Drawing for the job (mm, zero at the part's lowest x, y, z). Give positions to 0.01 mm unless a question says otherwise; leave off trailing zeros. Write each loop counter-clockwise with the first axis right and the second up, starting at its lowest first coordinate (ties: lowest second). Pieces come first, ordered by that corner, then holes.
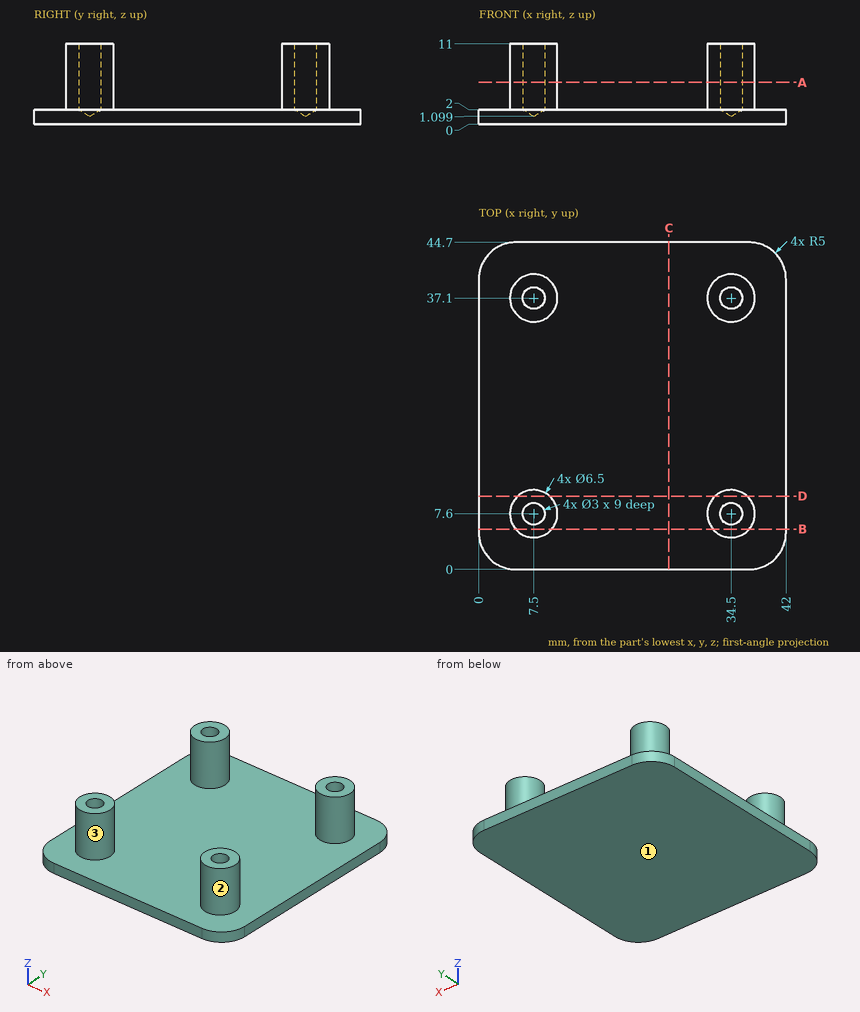
1. Probe probe 1 along Y at (x, z) = (34.5, 4.5); probe 2 along Z at (x, y) = (32.5, 24.5); probe 3 along X at (y, z) = (5, 4.5). List the from-to ranges inside material, lowest first.
Calculated:
probe 1: y = 4.35 to 6.1, 9.1 to 10.85, 33.85 to 35.6, 38.6 to 40.35
probe 2: z = 0 to 2
probe 3: x = 5.55 to 9.45, 32.55 to 36.45
2. Pull direction Y, two halves, no side cores. Call the marked faces 1, 2 and 3: +Y half, -Y half, draft (parallel to the pull), parting line (faces both ways), or undercut.
Calculated:
face 1: draft
face 2: undercut
face 3: undercut
3. Slice it at D-D, the plane y = 10. Write the cut outline in (x, z).
Calculated:
outline: (0, 0) - (42, 0) - (42, 2) - (36.69, 2) - (36.69, 11) - (32.31, 11) - (32.31, 2) - (9.69, 2) - (9.69, 11) - (5.31, 11) - (5.31, 2) - (0, 2) - close
4. Slice it at C-C, the plane x = 26. Write the cut outline in (y, z).
Calculated:
outline: (0, 0) - (44.7, 0) - (44.7, 2) - (0, 2) - close
5. Slice it at A-A, the plane z = 5.75. Write the cut outline in (x, y).
Calculated:
outline: circle Ø6.5 at (7.5, 7.6); circle Ø6.5 at (7.5, 37.1); circle Ø6.5 at (34.5, 7.6); circle Ø6.5 at (34.5, 37.1); hole circle Ø3 at (7.5, 7.6); hole circle Ø3 at (7.5, 37.1); hole circle Ø3 at (34.5, 7.6); hole circle Ø3 at (34.5, 37.1)
6. Pin check, flat tips, straight feed: P1, Ø1.8, axis at x = 34.5, y = 37.1, coming from the +Z side; P2, Ø2, axis at x = 26.5, y = 22.5, coming from the +Z side; P3, Ø4, axis at x = 7.5, y = 37.1, coming from the -Z side; P4, Ø5, axis at y = 40, z = 6, coming from the +X side (1 decimal). Stop position of each tip, or through.
Calculated:
P1: stops at z = 1.64
P2: stops at z = 2
P3: stops at z = 0
P4: stops at x = 37.7
7. Slice it at B-B, the plane y = 5.5. Write the cut outline in (x, z), and give its area (3 significant figures).
Calculated:
outline: (0, 0) - (42, 0) - (42, 2) - (36.98, 2) - (36.98, 11) - (32.02, 11) - (32.02, 2) - (9.98, 2) - (9.98, 11) - (5.02, 11) - (5.02, 2) - (0, 2) - close
area: 173 mm2
